Can you work these out from the model? Positions are in its coordinate system, mm. Coordinates: 2 decimals unless noted, no trailing zeros. Order: outer loops, then holes, each group sorted by start corner. A loop starts at its lowest first (then second) coordinate and runs counter-clockwise, first axis right, second up. Notation, with made-up numbers: (75.25, 36.25) -> (101.25, 36.25) arc R22 cw to (101.25, 75.25) -> close; hole circle Ø8 at (-15.5, -23). An arc over 180 degrees is marked (long way). Write item = value, one per line.
```python
from build123d import *

# Parameters (mm, degrees)
SKETCH1_W           = 150
SKETCH1_H           = 130
BOSS_EXTRUDE1_DEPTH = 600
SKETCH2_R           = 5
BOSS_EXTRUDE2_DEPTH = 200
SKETCH3_R           = 10
CUT_EXTRUDE1_DEPTH  = 0.1


with BuildPart() as part:
    # Sketch1 → Boss-Extrude1 (new body)
    with BuildSketch(Plane(origin=(0, 0, 0), x_dir=(0, 0, -1), z_dir=(1, 0, 0))):
        Rectangle(SKETCH1_W, SKETCH1_H)
    extrude(amount=BOSS_EXTRUDE1_DEPTH)

    # Sketch2 → Boss-Extrude2 (add)
    with BuildSketch(Plane.ZY):
        with Locations(Location((0, 0, 0), (0, 0, 180))):
            Circle(SKETCH2_R)
    extrude(amount=BOSS_EXTRUDE2_DEPTH)

    # Sketch3 → Cut-Extrude1 (cut)
    with BuildSketch(Plane(origin=(600, 0, 0), x_dir=(0, 0, -1), z_dir=(1, 0, 0))):
        Circle(SKETCH3_R)
    extrude(amount=-CUT_EXTRUDE1_DEPTH, mode=Mode.SUBTRACT)


solid = part.part
```
Item 1: If I drill on probe 1 along X at (y, z) = (-12, 56.5); probe 2 along Z at (x, y) = (-100, -0.5), over which ranges is the centre line in solid material (lowest first)?
A:
probe_1 = 0 to 600
probe_2 = -4.97 to 4.97
Item 2: I want a section at A-A, the plane y = -53. Please give me the cut outline in (x, z).
A:
outline = (0, -75) -> (600, -75) -> (600, 75) -> (0, 75) -> close
Item 3: I'm going to push flat-ended pins straight in: P1, Ø8, axis at y = -19, z = -9, coming from the -X side; P2, Ø6, axis at y = 3.5, z = -2, coming from the +X side. Where does each tip first touch, or does it pass through?
A:
P1 = 0
P2 = 599.9
Item 4: I want a section at B-B, the plane z = -18. Please give me the cut outline in (x, y).
A:
outline = (0, -65) -> (600, -65) -> (600, 65) -> (0, 65) -> close
